from build123d import *

# Parameters (mm, degrees)
F0_W      = 12
F0_H      = 10
F1_DEPTH  = 3.3
F2_SIZE   = 2
F3_R      = 3
F4_R      = 3
F5_R      = 1.75
F6_DEPTH  = 25
F7_R      = 2.5
F8_DEPTH  = 25
F9_R      = 4.25
F10_DEPTH = 25


with BuildPart() as f1:
    # F0 (on Top) → F1 (new body)
    with BuildSketch(Plane.XY):
        Polygon((15, -41), (15, 41), (3, 41), (-15, 41), (-15, -41), (-3, -41), align=None)
        with Locations((9, 46)):
            Rectangle(F0_W, F0_H)
        with Locations((-9, -46)):
            Rectangle(F0_W, F0_H)
    extrude(amount=F1_DEPTH)

    # F2
    f2_edges = [f1.edges().sort_by_distance(p)[0] for p in [
        (15, 51, 1.65),
        (3, 51, 1.65),
        (-15, -51, 1.65),
        (-3, -51, 1.65),
    ]]
    chamfer(f2_edges, length=F2_SIZE)

    # F3
    f3_edges = [f1.edges().sort_by_distance(p)[0] for p in [
        (3, 41, 1.65),
    ]]
    fillet(f3_edges, radius=F3_R)

    # F4
    f4_edges = [f1.edges().sort_by_distance(p)[0] for p in [
        (-3, -41, 1.65),
    ]]
    fillet(f4_edges, radius=F4_R)

    # F5 (on face) → F6 (cut)
    with BuildSketch(Plane.XY.offset(3.3)):
        with Locations((9, 46)):
            Circle(F5_R)
        with Locations((-9, -46)):
            Circle(F5_R)
    extrude(amount=-F6_DEPTH, mode=Mode.SUBTRACT)

    # F7 (on face) → F8 (cut)
    with BuildSketch(Plane.XY.offset(3.3)):
        with Locations((0, 26)):
            Circle(F7_R)
        with Locations((0, -26)):
            Circle(F7_R)
    extrude(amount=-F8_DEPTH, mode=Mode.SUBTRACT)

    # F9 (on face) → F10 (cut)
    with BuildSketch(Plane.XY.offset(3.3)):
        with Locations((0, 26)):
            Circle(F9_R)
        with Locations((0, -26)):
            Circle(F9_R)
        Circle(F9_R)
    extrude(amount=-F10_DEPTH, mode=Mode.SUBTRACT)


solid = f1.part
Could you check a few things on this model? Use its own coordinates, in mm. A direction names the side the tool comes from. Round coordinates to 2 decimals unless told otherwise and drop trailing zeros. Loops run counter-clockwise (first coordinate to the right, second up) from the corner with the lowest first, then second, coordinate; pieces in that order, holes last. Notation, with made-up numbers: (-18, 59) - (21, 59) arc R21 cw to (21, 65) - close; hole circle Ø9 at (20, -5.5). An arc over 180 degrees is marked (long way). Write item = value, one per line.
1) Imagine slicing it at D-D (x = -1). Please give me the cut outline in (y, z).
Computed:
outline = (-41.17, 0) - (-30.13, 0) - (-30.13, 3.3) - (-41.17, 3.3) - close; (-21.87, 0) - (-4.13, 0) - (-4.13, 3.3) - (-21.87, 3.3) - close; (4.13, 0) - (21.87, 0) - (21.87, 3.3) - (4.13, 3.3) - close; (30.13, 0) - (41, 0) - (41, 3.3) - (30.13, 3.3) - close
2) If we mould it in two halves opening along X, with no side actions, what happens to faces 4 (the cylindrical face through (-2.1, -41.86, 1.67)), 5 (the cylindrical face through (8.62, 44.29, 1.67)), 6 (the flat face through (-7, 1, 0))? For each: pulls with the +X half, pulls with the -X half, needs draft (parallel to the pull), parting line crosses it, or undercut.
Computed:
face_4 = pulls with the +X half
face_5 = undercut
face_6 = needs draft
3) Imagine slicing it at C-C (z = 0.95). Please give me the cut outline in (x, y), and give its area (3 significant figures).
Computed:
outline = (-15, -49) - (-13, -51) - (-5, -51) - (-3, -49) - (-3, -44) arc R3 cw to (0, -41) - (15, -41) - (15, 49) - (13, 51) - (5, 51) - (3, 49) - (3, 44) arc R3 cw to (0, 41) - (-15, 41) - close; hole circle Ø3.5 at (-9, -46); hole circle Ø8.5 at (0, -26); hole circle Ø8.5 at (0, 0); hole circle Ø8.5 at (0, 26); hole circle Ø3.5 at (9, 46)
area = 2,510 mm2
4) I need wall thicknesses on line 1 along Y through (x, z) = (-1.25, 0.75); line 2 along Y through (x, z) = (-0.75, 0.85); line 3 along Y through (x, z) = (9, 3.15). Which ranges of each line are inside material? Lowest first, please. Write a range as from..to.
Computed:
line_1 = -41.27..-30.06, -21.94..-4.06, 4.06..21.94, 30.06..41
line_2 = -41.1..-30.18, -21.82..-4.18, 4.18..21.82, 30.18..41
line_3 = -41..44.25, 47.75..51
5) On a 3-axis mill with a long thin cutter (end or side, diameter ignored), from which of +Z, -Z, +X, -X, +Y, -Y can I reach the whole of each face in a straight line? I mean faces 1 (the cylindrical face through (2.285, 3.584, 1.673)), 2 (the flat face through (3, 46, 2)), 3 (the flat face through (-3, -47, 2)). Say none if no direction works.
Computed:
face_1 = +Z, -Z
face_2 = +Z, -Z, -X, +Y
face_3 = +Z, -Z, +X, -Y
6) Imagine slicing it at A-A (y = -46). Please give me the cut outline in (x, z), and give its area (4 significant figures).
Computed:
outline = (-15, 0) - (-10.75, 0) - (-10.75, 3.3) - (-15, 3.3) - close; (-7.25, 0) - (-3, 0) - (-3, 3.3) - (-7.25, 3.3) - close
area = 28.05 mm2
7) Imagine slicing it at B-B (x = -9). Please give me the cut outline in (y, z).
Computed:
outline = (-51, 0) - (-47.75, 0) - (-47.75, 3.3) - (-51, 3.3) - close; (-44.25, 0) - (41, 0) - (41, 3.3) - (-44.25, 3.3) - close
8) I'm going to push flat-ended pins straight in: P1, Ø2, axis at x = 9, y = 46, coming from the +Z side; P2, Ø1, axis at y = 47.5, z = 1, coming from the -X side; P3, Ø1, axis at x = -4, z = 2, coming from the +Y side. Where does each tip first touch, or does it pass through?
Computed:
P1 = through
P2 = 3
P3 = 41
